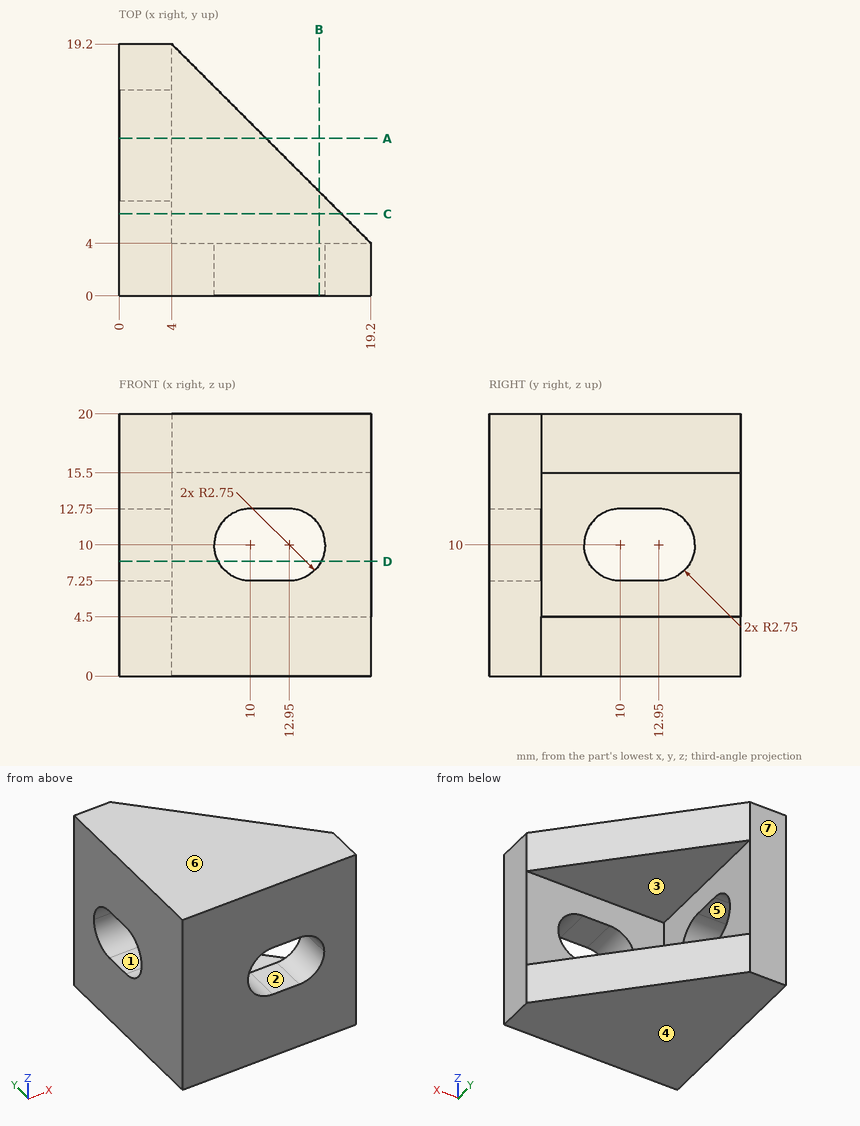
Can you work these out from the drawing? Everything is in mm from the part's minimum corner. A direction names the side the tool comes from. Give positions to 0.01 mm unless a question says otherwise; leave off trailing zeros. Loops run counter-clockwise (first coordinate to the right, second up) from the corner with the lowest first, then second, coordinate; pieces in that order, holes last. Notation, with made-up numbers: (63, -31.75) - (82, -31.75) arc R21 ccw to (82, -14.75) - close; hole circle Ø4 at (31.5, 66.25). An arc over 180 degrees is marked (long way). Answer as a JSON object with one key per item and string values.
Q1. Will these pins go through, and if not, where does the flat tip stop? P1, Ø3, axis at y = 10, z = 11.5, coming from the +X side; P2, Ø5.5, axis at x = 9, z = 8, coming from the +Y side; P3, Ø1, axis at x = 15, y = 9.5, coming from the +Z side.
Geometry says:
{"P1": "x = 4", "P2": "y = 4", "P3": "through"}
Q2. If I drill on L1, parallel to Z at x = 13, y = 5; L2, parallel to Y at x = 17.75, z = 13.5, over which ranges is the centre line in solid material (lowest first)?
Geometry says:
{"L1": "0 to 4.5, 15.5 to 20", "L2": "0 to 4"}
Q3. Which directions (+Z, -Z, +X, -X, +Y, -Y) give clear straight access to the entire face, cutting with the end or side of a thin tool? Please do the marked faces 1, 2 and 3.
Geometry says:
{"face 1": "+X, -X", "face 2": "+Y, -Y", "face 3": "+X, +Y"}
Q4. Imagine slicing it at B-B on x = 15.25. Write out the boundary of the cut face in (y, z), plus the area to 3 significant figures.
Geometry says:
{"outline": "(0, 0) - (7.95, 0) - (7.95, 4.5) - (4, 4.5) - (4, 8.49) - (0, 8.49) - close; (0, 11.51) - (4, 11.51) - (4, 15.5) - (7.95, 15.5) - (7.95, 20) - (0, 20) - close", "area": "103 mm²"}
Q5. Imagine slicing it at A-A on y = 12. Write out the boundary of the cut face in (x, z), plus the area to 3 significant figures.
Geometry says:
{"outline": "(0, 0) - (11.2, 0) - (11.2, 4.5) - (4, 4.5) - (4, 7.25) - (0, 7.25) - close; (0, 12.75) - (4, 12.75) - (4, 15.5) - (11.2, 15.5) - (11.2, 20) - (0, 20) - close", "area": "123 mm²"}
Q6. Imagine slicing it at D-D on z = 8.75. Write out the boundary of the cut face in (x, y), plus the area to 3 significant figures.
Geometry says:
{"outline": "(0, 0) - (7.55, 0) - (7.55, 4) - (4, 4) - (4, 7.55) - (0, 7.55) - close; (0, 15.4) - (4, 15.4) - (4, 19.2) - (0, 19.2) - close; (15.4, 0) - (19.2, 0) - (19.2, 4) - (15.4, 4) - close", "area": "74.8 mm²"}
Q7. Imagine slicing it at C-C on y = 6.25. Write out the boundary of the cut face in (x, z).
Geometry says:
{"outline": "(0, 0) - (16.95, 0) - (16.95, 4.5) - (4, 4.5) - (4, 15.5) - (16.95, 15.5) - (16.95, 20) - (0, 20) - close"}
Q8. If we mould it in two halves opening along Z, with no side actions, what happens to the marked faces 4, 5, 6 and 7? For each: pulls with the +Z half, pulls with the -Z half, needs draft (parallel to the pull), parting line crosses it, or undercut.
Geometry says:
{"face 4": "pulls with the -Z half", "face 5": "undercut", "face 6": "pulls with the +Z half", "face 7": "needs draft"}
